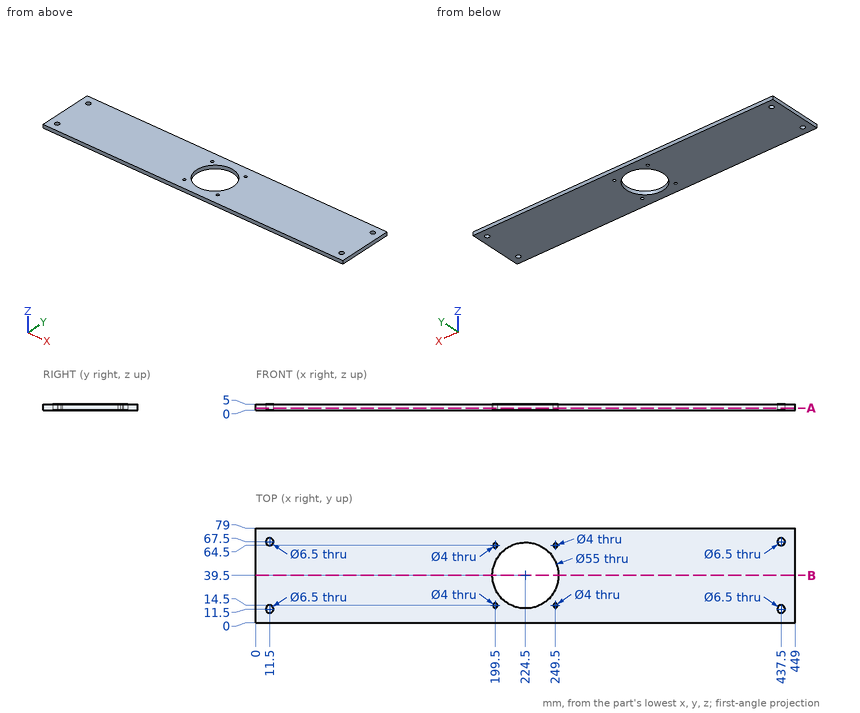
Answer from the drawing. Dimensions are ordinates in mm from the lowest x, y and z of the part. Give positions to 0.01 mm unless a question says otherwise; leave off trailing zeros. Order: outer loops, then holes, each group sorted by start corner. A loop starts at its lowest first (then second) coordinate and runs counter-clockwise, first axis right, second up.
(1) Find section B-B (y = 39.5). Give the vertices of the cut face in (x, z), plus the area to 3 significant figures.
(2) Find section A-A (z = 1.6). Give the number of separate pieces and of enclosed holes in the cut face, plus the area to 3 significant figures.
(3) Given pin 1 (5 mm diameter, centred on x = 249.5, y = 14.5, fed in from -Z); pin 2 (2 mm diameter, centred on x = 207, y = 20, fed in from +Z), each flat-ended and moving along its own axis, determine where each tip first touches the part or whether it passes through.
(4) Straight lines are drawn through the part: L1, parallel to Y at x = 437.5, z = 3.85; L2, parallel to Y at x = 229.5, z = 2.75; L3, parallel to Y at x = 199.5, z = 2. For each, find the intervals that lie inside material, in ascending order.
Result sheet:
1. outline: (0, 0) - (197, 0) - (197, 5) - (0, 5) - close; (252, 0) - (449, 0) - (449, 5) - (252, 5) - close
1. area: 1,970 mm2
2. separate pieces: 1
2. enclosed holes: 9
2. area: 32,900 mm2
3. pin 1: stops at z = 0
3. pin 2: passes through
4. L1: y = 0 to 8.25, 14.75 to 64.25, 70.75 to 79
4. L2: y = 0 to 12.46, 66.54 to 79
4. L3: y = 0 to 12.5, 16.5 to 28.04, 50.96 to 62.5, 66.5 to 79
